from build123d import *

# Parameters (mm, degrees)
PAD001_DEPTH         = 13
SKETCH004_W          = 27.5
SKETCH004_H          = 20
POCKET_DEPTH         = 4.5
SKETCH005_R          = 3
HOLE_DEPTH           = 25
POCKET001_DEPTH      = 42.001
POCKET001_DEPTH_BACK = 16.001


with BuildPart() as part:
    # Sketch003 (on CopyRevolution) → Pad001 (new body)
    with BuildSketch(Plane(origin=(0, 0, 100), x_dir=(0, -1, 0), z_dir=(0, 0, 1))):
        with BuildLine():
            Line((-55, -13), (-55, 13))
            Line((-55, 13), (-37, 13))
            ThreePointArc((-37, 13), (-28.354779, 14.789176), (-21.129846, 19.862769))
            ThreePointArc((-21.129846, -19.862769), (29, 0), (-21.129846, 19.862769))
            ThreePointArc((-21.129846, -19.862769), (-28.354779, -14.789176), (-37, -13))
            Line((-37, -13), (-55, -13))
        make_face()
    extrude(amount=PAD001_DEPTH)

    # Sketch004 (on Face8 of Pad001) → Pocket (cut)
    with BuildSketch(Plane(origin=(0, 0, 113), x_dir=(0, -1, 0), z_dir=(0, 0, 1))):
        with Locations((-41.25, 0)):
            Rectangle(SKETCH004_W, SKETCH004_H)
    extrude(amount=-POCKET_DEPTH, mode=Mode.SUBTRACT)

    # Sketch005 (on Face12 of Pocket) → Hole (cut)
    with BuildSketch(Plane(origin=(0, 0, 108.5), x_dir=(0, -1, 0), z_dir=(0, 0, 1))):
        with Locations((-45.05, 0)):
            Circle(SKETCH005_R)
    extrude(amount=-HOLE_DEPTH, mode=Mode.SUBTRACT)

    # Sketch006 (on Face8 of Hole) → Pocket001 (cut, two sides)
    with BuildSketch(Plane.YZ.offset(13)) as pocket001_sk:
        Polygon((55, 107), (49, 105), (30.5, 105), (27.5, 100), (55, 100), align=None)
    extrude(amount=-POCKET001_DEPTH, mode=Mode.SUBTRACT)
    extrude(pocket001_sk.sketch, amount=POCKET001_DEPTH_BACK, mode=Mode.SUBTRACT)


solid = part.part
Can you work these out from the model? Positions are in its coordinate system, mm. A direction names the side the tool comes from. Coordinates: 2 decimals unless noted, no trailing zeros. Loops run counter-clockwise (first coordinate to the right, second up) from the corner with the lowest first, then second, coordinate; pieces in that order, holes last. Notation, with made-up numbers: M -17,53 L 15,53 A18 cw 15,60 Z; hole C 73,-4 d10. An arc over 180 degrees is marked long. Return JSON: item names as keys, results as strings. Group by question number.
Item 1: I'm going to push flat-ended pins straight in: pin 1 Ø6.5 at (y, z) = (46.5, 109.5) entering from -X; pin 2 Ø4 at (y, z) = (45, 104.5) entering from +X; pin 3 Ø6 at (y, z) = (5.5, 106.5) entering from -X. Where does each tip first touch, or does it pass through?
Item 2: Thinking about a two-plate mould opening in X: for faces 4 (the flat face through (0, 52, 106)), 5 (the cylindrical face through (-0.969, -28.984, 106.409)), 6 (the cylindrical face through (0.132, 48.047, 106.774)), which applies, released by +X, released by -X, zero draft, split by the parting line, or undercut?
Item 3: Imagine slicing it at B-B (x = 0). Please give me the cut outline in (y, z), and give its area (3 significant figures).
Item 4: Imagine slicing it at A-A (y = 45.05). Please give me the cut outline in (x, z), and give its area (3 significant figures).
Item 5: If I drill on L1, parallel to X at y = 45.05, z = 107.8; L2, parallel to X at y = 43, z = 110.25; L3, parallel to Y at x = -6.5, z = 104, over which ranges is the centre line in solid material (lowest first)? Write a range as from..to.
Item 6: Imagine slicing it at C-C (x = -7.5). Please give me the cut outline in (y, z), and give its area (3 significant figures).
Item 7: Imagine slicing it at D-D (y = 33). Please give me the cut outline in (x, z).
Item 8: On a 3-axis mill with a long thin cutter (end or side, diameter ignored), from which of +Z, -Z, +X, -X, +Y, -Y can I reach the whole of each face in a straight line? I mean faces 1 (the flat face through (0, 27.5, 111)), 2 (the flat face through (13, 46, 109)), 3 (the flat face through (0, 40, 105)). Say none if no direction works.
Verdict:
{
 "1": {"pin 1": "stops at x = -13", "pin 2": "stops at x = 13", "pin 3": "stops at x = -28.89"},
 "2": {"face 4": "zero draft", "face 5": "split by the parting line", "face 6": "undercut"},
 "3": {"outline": "M -29,100 L 27.5,100 L 30.5,105 L 42.05,105 L 42.05,108.5 L 27.5,108.5 L 27.5,113 L -29,113 Z; M 48.05,105 L 49,105 L 55,107 L 55,108.5 L 48.05,108.5 Z", "area": "811 mm^2"},
 "4": {"outline": "M -13,105 L -3,105 L -3,108.5 L -10,108.5 L -10,113 L -13,113 Z; M 3,105 L 13,105 L 13,113 L 10,113 L 10,108.5 L 3,108.5 Z", "area": "97.0 mm^2"},
 "5": {"L1": "x = -13..-3, 3..13", "L2": "x = -13..-10, 10..13", "L3": "y = -28.26..29.9"},
 "6": {"outline": "M -28.01,100 L 27.5,100 L 30.5,105 L 49,105 L 55,107 L 55,108.5 L 27.5,108.5 L 27.5,113 L -28.01,113 Z", "area": "819 mm^2"},
 "7": {"outline": "M -13.37,105 L 13.37,105 L 13.37,113 L 10,113 L 10,108.5 L -10,108.5 L -10,113 L -13.37,113 Z"},
 "8": {"face 1": "+Z, +Y", "face 2": "+Z, -Z, +X, +Y", "face 3": "-Z, +X, -X, +Y"}
}
